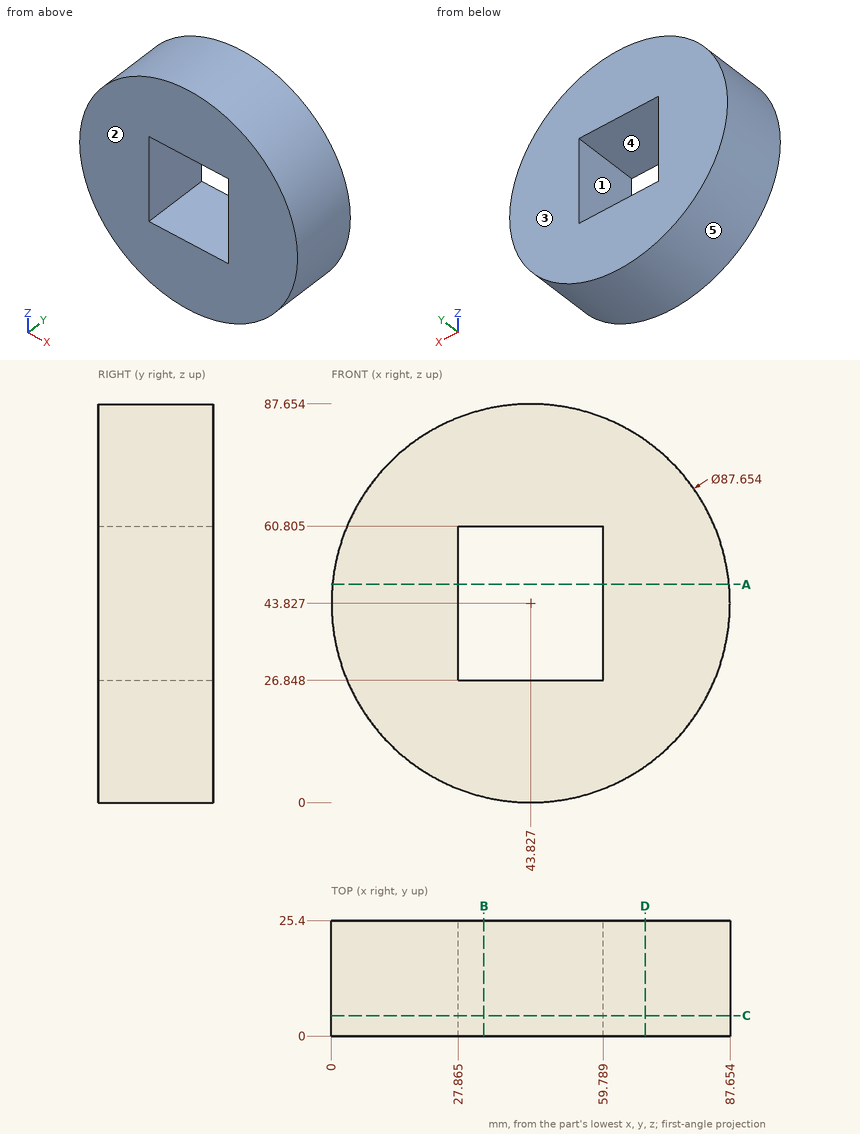
The drawing under review shows one solid part. Ordinate dimensions are in mm from its lowest x, y, z. A direction names the side the tool comes from. Coordinates: 2 decimals unless noted, no trailing zeros. Write each loop counter-clockwise with the first axis right and the second up, starting at its lowest first coordinate (ties: lowest second). Pieces come first, ordered by that corner, then holes. Notation, with made-up numbers: (-27, 35.25) -> (26, 35.25) arc R15 ccw to (26, 50.25) -> close; hole circle Ø7 at (55.5, 14.25). An arc over 180 degrees is marked (long way). Write each question's results on one line, items separated by ' | '. Start each with the question number.
1) Insertion check: pin 1 (2 mm diameter, centred on x = 55.5, y = 21.5, fed in from -Z); pin 2 (7.5 mm diameter, centred on x = 42, y = 13, fed in from +Z); pin 3 (12 mm diameter, centred on x = 53, y = 23, fed in from +Z). Each pin has a flat end and moves straight along its axis. Give the tip position at first contact, or say it passes through.
2) For the marked faces 1 and 2, list the 3-axis set-ups (+Z, -Z, +X, -X, +Y, -Y) from which the entire face can be reached by the end or side of a thin tool; tool diameter is ignored.
3) Consider section A-A (z = 48). Write out the cut boundary in (x, y) (1 decimal).
4) Wall thickness on L1, parallel to X at y = 17.75, z = 32 (1 decimal); L2, parallel to Z at x = 36.5, y = 21.5 (1 decimal); L3, parallel to Z at x = 41, y = 21.75 (1 decimal): over which ranges is each line inside the solid? List them lowest first. Write a range as [from, to].
5) Consider section C-C (y = 4.5). Write out the cut boundary in (x, z) (1 decimal), plus the area to 3 significant figures.
6) Consider section B-B (x = 33.5). Write out the cut boundary in (y, z) (1 decimal).
7) Consider section D-D (x = 69). Write out the cut boundary in (y, z), plus the area to 3 significant figures.
8) The part is to be moulded in two halves that separate along X. For the marked faces 3, 4 and 5, say which applies: +X half, -X half, draft (parallel to the pull), parting line (faces both ways), or undercut.
Geometry says:
1) pin 1: z = 1.32 | pin 2: z = 87.65 | pin 3: z = 87.54
2) face 1: +Y, -Y | face 2: +Z, -Z, +X, -X, -Y
3) outline: (0.2, 0) -> (27.9, 0) -> (27.9, 25.4) -> (0.2, 25.4) -> close; (59.8, 0) -> (87.5, 0) -> (87.5, 25.4) -> (59.8, 25.4) -> close
4) L1: [1.6, 27.9], [59.8, 86] | L2: [0.6, 26.8], [60.8, 87] | L3: [0.1, 26.8], [60.8, 87.6]
5) outline: circle Ø87.7 at (43.8, 43.8); hole (27.9, 26.8) -> (59.8, 26.8) -> (59.8, 60.8) -> (27.9, 60.8) -> close | area: 4,950 mm^2
6) outline: (0, 1.2) -> (25.4, 1.2) -> (25.4, 26.8) -> (0, 26.8) -> close; (0, 60.8) -> (25.4, 60.8) -> (25.4, 86.4) -> (0, 86.4) -> close
7) outline: (0, 7.95) -> (25.4, 7.95) -> (25.4, 79.7) -> (0, 79.7) -> close | area: 1,820 mm^2
8) face 3: draft | face 4: undercut | face 5: parting line
